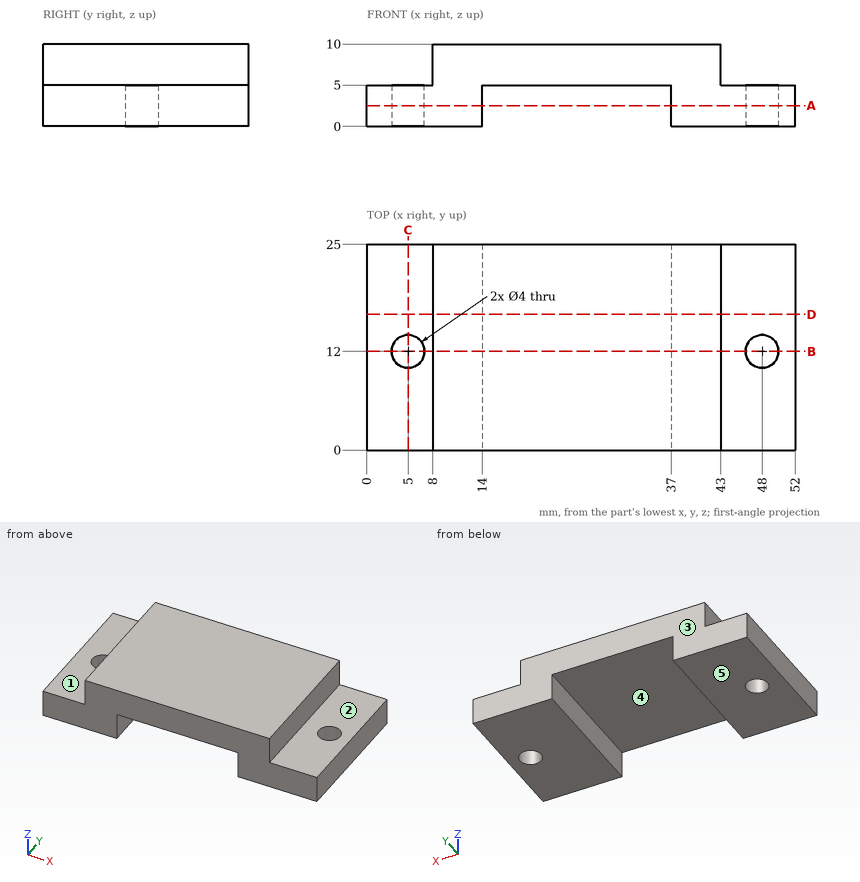
Geometry: see drawing. Coordinates: mm, zero at the bounding-box minimum. A direction names the side the tool comes from. Give positions to 0.01 mm unless a question says otherwise; leave off trailing zeros. Write each loop counter-clockwise with the first axis right and the second up, starting at its lowest first coordinate (ties: lowest second). Pieces come first, ordered by that corner, then holes. Notation, with made-up numbers: M -35.75,2.5 L -7.75,2.5 A13 ccw -7.75,24.5 Z; hole C -13,24.5 d3. An arc over 180 degrees is marked long. Answer in a Markdown table with one row per item. Add a question column.
(1) Mould query, pull axis X, two halves, no side actions, for the marked faces 4 and 5. Classes: +X half, -X half, draft (parallel to the pull), parting line (faces both ways), or undercut.
(2) Ray query, line 1 (X direction, y = 21.5, z = 2); line 2 (Y direction, x = 48, z = 2.2); line 3 (Z direction, x = 20.5, y = 22.25). Return the intervals inside material, ascending.
(3) Section B-B on y = 12. Return loops of the section in (x, z), and give its area (3 significant figures).
(4) Section A-A on z = 2.5. Return loops of the section in (x, y), and give its area (3 significant figures).
(5) Reachability of the marked faces 1, 2 and 3 from +Z, -Z, +X, -X, +Y, -Y: full face, straight path, thin tool, end or side. Return the list, or none.
(6) Section C-C on x = 5. Return loops of the section in (y, z).
(7) First-contact query: pin 1 (4.5 mm diameter, centred on x = 48, y = 12, fed in from -Z); pin 2 (7 mm diameter, centred on x = 21.5, y = 16, fed in from -Z); pin 3 (4 mm diameter, centred on y = 12, z = 7.5, fed in from -X); pin 4 (2.5 mm diameter, centred on x = 47.5, y = 18, fed in from +Z). Flat tips, straight axial feed; report the tip coordinate or a pass-through.
(8) Section D-D on y = 16.5. Return loops of the section in (x, z), and give its area (3 significant figures).
Result set:
| question | item | result |
|---|---|---|
| 1 | face 4 | undercut |
| 1 | face 5 | draft |
| 2 | line 1 | x = 0 to 14, 37 to 52 |
| 2 | line 2 | y = 0 to 10, 14 to 25 |
| 2 | line 3 | z = 5 to 10 |
| 3 | outline | M 0,0 L 3,0 L 3,5 L 0,5 Z; M 7,0 L 14,0 L 14,5 L 37,5 L 37,0 L 46,0 L 46,5 L 43,5 L 43,10 L 8,10 L 8,5 L 7,5 Z; M 50,0 L 52,0 L 52,5 L 50,5 Z |
| 3 | area | 280 mm^2 |
| 4 | outline | M 0,0 L 14,0 L 14,25 L 0,25 Z; M 37,0 L 52,0 L 52,25 L 37,25 Z; hole C 5,12 d4; hole C 48,12 d4 |
| 4 | area | 700 mm^2 |
| 5 | face 1 | +Z, -X, +Y, -Y |
| 5 | face 2 | +Z, +X, +Y, -Y |
| 5 | face 3 | +Z, -Z, +X, -X, +Y |
| 6 | outline | M 0,0 L 10,0 L 10,5 L 0,5 Z; M 14,0 L 25,0 L 25,5 L 14,5 Z |
| 7 | pin 1 | stops at z = 0 |
| 7 | pin 2 | stops at z = 5 |
| 7 | pin 3 | stops at x = 8 |
| 7 | pin 4 | stops at z = 5 |
| 8 | outline | M 0,0 L 14,0 L 14,5 L 37,5 L 37,0 L 52,0 L 52,5 L 43,5 L 43,10 L 8,10 L 8,5 L 0,5 Z |
| 8 | area | 320 mm^2 |
